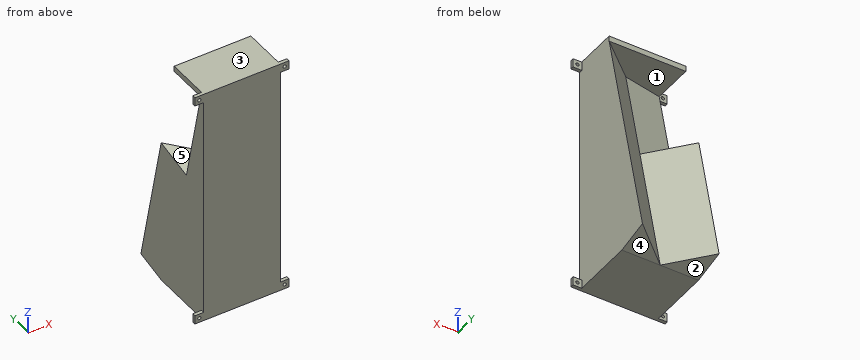
from build123d import *

# Parameters (mm, degrees)
SKETCH3_W           = 220
SKETCH3_H           = 10
BOSS_EXTRUDE2_DEPTH = 70
BOSS_EXTRUDE3_DEPTH = 130
BOSS_EXTRUDE4_DEPTH = 225
CUT_EXTRUDE1_START  = -227.161631
CUT_EXTRUDE1_DEPTH  = 97.161631
BOSS_EXTRUDE5_REACH = 249.52
SKETCH9_W           = 5
SKETCH9_H           = 41.901402289
SKETCH10_W          = 13.70856438
SKETCH10_H          = 41.94949396
CUT_EXTRUDE2_DEPTH  = 248.520249593
SKETCH11_W          = 8
SKETCH11_H          = 8
SKETCH11_R          = 1.5
BOSS_EXTRUDE6_DEPTH = 3


with BuildPart() as part:
    # Sketch3 → Boss-Extrude2 (new body)
    with BuildSketch(Plane(origin=(0, 0, 0), x_dir=(0, 0, -1), z_dir=(1, 0, 0))):
        Polygon((220, 10), (220, 60), (0, 10), align=None)
        with Locations((110, 5)):
            Rectangle(SKETCH3_W, SKETCH3_H)
    extrude(amount=BOSS_EXTRUDE2_DEPTH)

    # Sketch4 → Boss-Extrude3 (add)
    with BuildSketch(Plane(origin=(0, 50.491159136, -222.161100196), x_dir=(-1, 0, 0), z_dir=(0, 0.22162110358896814, -0.9751328557914598))):
        Polygon((-70, 39.751328558), (-70, 9.751328558), (-35, 9.751328558), align=None)
        Polygon((0, 39.751328558), (-35, 9.751328558), (0, 9.751328558), align=None)
    extrude(amount=-BOSS_EXTRUDE3_DEPTH)

    # Sketch4<3> → Boss-Extrude4 (add)
    with BuildSketch(Plane(origin=(0, 50.491159136, -222.161100196), x_dir=(-1, 0, 0), z_dir=(0, 0.22162110358896814, -0.9751328557914598))):
        Polygon((-70, 39.751328558), (-70, 9.751328558), (-35, 9.751328558), align=None)
    extrude(amount=-BOSS_EXTRUDE4_DEPTH)

    # Sketch8 → Cut-Extrude1 (cut)
    with BuildSketch(Plane(origin=(0, 50.491159136, -222.161100196), x_dir=(-1, 0, 0), z_dir=(0, 0.22162110358896814, -0.9751328557914598)).offset(CUT_EXTRUDE1_START)):
        Polygon((-35, 9.751328558), (0, 2.925398567), (0, 9.751328558), align=None)
    extrude(amount=CUT_EXTRUDE1_DEPTH, mode=Mode.SUBTRACT)

    # Boss-Extrude5: up to this face of the body (flat: up to its plane)
    boss_extrude5_end = Plane(part.part.faces().sort_by_distance((70, 34.124937216, -122.542284952))[0])
    # Sketch9 → Boss-Extrude5 (add, up to the picked face)
    with BuildSketch(Plane.ZY, mode=Mode.PRIVATE) as boss_extrude5_sk1:
        with Locations((-2.5, 20.950701145)):
            Rectangle(SKETCH9_W, SKETCH9_H)
    boss_extrude5_tool1 = split(extrude(boss_extrude5_sk1.sketch, amount=-BOSS_EXTRUDE5_REACH, mode=Mode.PRIVATE), bisect_by=boss_extrude5_end, keep=Keep.BOTH, mode=Mode.PRIVATE)
    add(boss_extrude5_tool1.solids().sort_by(Axis((0, 20.950701, -2.5), (1, 0, 0)))[0])

    # Sketch10 → Cut-Extrude2 (cut, through all)
    with BuildSketch(Plane.ZY):
        with Locations((6.85428219, 20.97474698)):
            Rectangle(SKETCH10_W, SKETCH10_H)
    extrude(amount=-CUT_EXTRUDE2_DEPTH, mode=Mode.SUBTRACT)

    # Sketch11 → Boss-Extrude6 (add)
    # profile 1 of 4: a face of its own
    with BuildSketch(Plane(origin=(0, 0, 0), x_dir=(1, 0, 0), z_dir=(0, 1, 0))):
        with Locations((-4, 216)):
            Rectangle(SKETCH11_W, SKETCH11_H)
        with Locations(Location((-4, 216, 0), (0, 0, 270))):
            Circle(SKETCH11_R, mode=Mode.SUBTRACT)
    # profile 2 of 4: a face of its own
    with BuildSketch(Plane(origin=(0, 0, 0), x_dir=(1, 0, 0), z_dir=(0, 1, 0))):
        with Locations((74, 216)):
            Rectangle(SKETCH11_W, SKETCH11_H)
        with Locations(Location((74, 216, 0), (0, 0, 270))):
            Circle(SKETCH11_R, mode=Mode.SUBTRACT)
    # profile 3 of 4: a face of its own
    with BuildSketch(Plane(origin=(0, 0, 0), x_dir=(1, 0, 0), z_dir=(0, 1, 0))):
        with Locations((-4, 4)):
            Rectangle(SKETCH11_W, SKETCH11_H)
        with Locations(Location((-4, 4, 0), (0, 0, 270))):
            Circle(SKETCH11_R, mode=Mode.SUBTRACT)
    # profile 4 of 4: a face of its own
    with BuildSketch(Plane(origin=(0, 0, 0), x_dir=(1, 0, 0), z_dir=(0, 1, 0))):
        with Locations((74, 4)):
            Rectangle(SKETCH11_W, SKETCH11_H)
        with Locations(Location((74, 4, 0), (0, 0, 270))):
            Circle(SKETCH11_R, mode=Mode.SUBTRACT)
    extrude(amount=BOSS_EXTRUDE6_DEPTH)


solid = part.part
Read the model definition and answer for the solid it produces. Units are mm, in the model's axes. Face numbers are marked on the shaded views. A direction names the side the tool comes from. Round coordinates to 2 decimals unless told otherwise and drop trailing zeros. Order: outer loops, then holes, each group sorted by start corner. A loop starts at its lowest first (then second) coordinate and runs counter-clockwise, first axis right, second up. Notation, with made-up numbers: (-3, 86.5) - (13, 86.5) arc R10 cw to (13, 95.5) - close; hole circle Ø1 at (16.5, 55.5). An arc over 180 degrees is marked (long way). Use one line per item in the form item = value. Start each with the question number.
(1) The part is cut by section B-B (x = 20.5). Give the vertices of the cut face in (y, z), then the cut area to 3 significant figures.
(2) The part is cut by section C-C (z = -149). Give the vertices of the cut face in (x, y), then the cut area to 3 significant figures.
(3) Find the intervals of material crossed by line 1 along Z through (x, y) = (74, 1.15); line 2 along X through (y, z) = (1.95, -216); line 3 along X through (y, z) = (17, -189.5), in increasing order. Write a range as from..to.
(4) Determine the mould class of the marked faces 1, 2 and 3 for opening direction Z: +Z half, -Z half, draft (parallel to the pull), parting line (faces both ways), or undercut.
(5) The part is cut by section A-A (y = 80.5). Give the vertices of the cut face in (x, z).
(6) Flat-ended cylindrical pins translate along their axes: pin 1 Ø2 at (x, z) = (30, -30.5) entering from +Y; pin 2 Ø5 at (x, z) = (45.5, -169.5) entering from +Y; pin 3 Ø1 at (x, z) = (26, -43) entering from +Y; pin 4 Ø2.5 at (x, z) = (74, -216) entering from +Y. Find the tip coordinate at first contact, or state that the pin passes through.
(7) For the marked faces 4 and 5, determine the directions among +Z, -Z, +X, -X, +Y, -Y from which every point of the face is accessible in a straight line to the end or side of a thin tool.
(8) The part is cut by section D-D (y = 17). Give the vertices of the cut face in (x, z), then the cut area to 3 significant figures.
Checked values:
q1.outline = (0, -220) - (60, -220) - (72.12, -217.25) - (43.31, -90.48) - (28.43, -93.86) - (8.24, -5) - (41.9, -5) - (41.9, 0) - (0, 0) - close
q1.area = 9,220 mm^2
q2.outline = (0, 0) - (70, 0) - (70, 74.63) - (35, 43.86) - (0, 74.63) - close
q2.area = 4,150 mm^2
q3.line_1 = -220..-217.5, -214.5..-212, -8..-5.5, -2.5..0
q3.line_2 = -8..-5.5, -2.5..72.5, 75.5..78
q3.line_3 = 0..70
q4.face_1 = undercut
q4.face_2 = -Z half
q4.face_3 = +Z half
q5.outline = (0, -215.34) - (10.47, -215.34) - (0, -174.83) - close; (59.53, -215.34) - (70, -215.34) - (70, -174.83) - close
q6.pin_1 = 16.23
q6.pin_2 = 60.02
q6.pin_3 = 18.12
q6.pin_4 = through
q7.face_4 = -Z, +X, -X, +Y
q7.face_5 = -X
q8.outline = (0, -220) - (70, -220) - (70, 0) - (0, 0) - (0, -5) - (41.67, -5) - (35, -30.8) - (0, -61.6) - close
q8.area = 13,900 mm^2
